from build123d import *

# Parameters (mm, degrees)
F2_R     = 12.7
F3_DEPTH = 7.62


with BuildPart() as f1:
    # F0 (on Front) → F1 (revolve)
    with BuildSketch(Plane.XZ):
        with BuildLine():
            Line((15.875, 35.306), (3.175, 35.306))
            Line((3.175, 35.306), (3.175, 0))
            Line((3.175, 0), (19.05, 0))
            Line((19.05, 0), (19.05, 3.175))
            ThreePointArc((19.05, 3.175), (16.685437, 8.304086), (15.875, 13.893529))
            Line((15.875, 13.893529), (15.875, 35.306))
        make_face()
    revolve(axis=Axis((0, 0, 26.439369), (0, 0, 1)))

    # F2 (on face) → F3 (cut)
    with BuildSketch(Plane.XY.offset(35.306)):
        Circle(F2_R)
    extrude(amount=-F3_DEPTH, mode=Mode.SUBTRACT)


solid = f1.part
Here's how the part is built. I have some questions about the finished solid (model axes, mm). A direction names the side the tool comes from. Coordinates: 2 decimals unless noted, no trailing zeros. Write each loop counter-clockwise with the first axis right and the second up, starting at its lowest first coordinate (ties: lowest second). Pieces come first, ordered by that corner, then holes.
Item 1: I want a section at C-C on z = 12. Write out the boundary of the cut face in (x, y) (3 decimals).
Item 2: If we mould it in two halves opening along Y, with no side actions, what happens to faces 3 (the flat face through (-7, 11, 35.306)), 4 (the flat face through (3, -3, 27.686)), 5 (the cylindrical face through (-3.441, -15.497, 24.75))? For each: +Y half, -Y half, draft (parallel to the pull), parting line (faces both ways), or undercut.
Item 3: If I drill on line 1 (Y direction, x = 0, z = 14) (3 decimals); line 2 (Y direction, x = 0, z = 31.75) (3 decimals); line 3 (Z direction, x = 6, y = 9), over which ranges is the centre line in solid material (lowest first)?
Item 4: On a 3-axis mill with a long thin cutter (end or side, diameter ignored), from which of +Z, -Z, +X, -X, +Y, -Y can I reach the whole of each face in a straight line? I mean faces 1 (the flat face through (-4, 0, 0)), 2 (the cylindrical face through (-2.75, -12.4, 31.55)). Say none if no direction works.
Item 5: Will these pins go through, and if not, where does the flat tip stop? pin 1 (12 mm diameter, centred on y = -4.5, z = 20, fed in from -X) (3 decimals); pin 2 (4 mm diameter, centred on x = 0.5, y = 6.5, fed in from +Z); pin 3 (6 mm diameter, centred on x = -12.5, z = 9, fed in from -Y); pin 4 (15 mm diameter, centred on x = 0, y = 0, fed in from -Z).
Item 6: I want a section at A-A on y = 0. Write out the boundary of the cut face in (x, z) (3 decimals).
Findings below:
1. outline: circle Ø31.933 at (0, 0); hole circle Ø6.35 at (0, 0)
2. face 3: draft
2. face 4: undercut
2. face 5: parting line
3. line 1: y = -15.875 to -3.175, 3.175 to 15.875
3. line 2: y = -15.875 to -12.7, 12.7 to 15.875
3. line 3: z = 0 to 27.69
4. face 1: -Z, +X, -X, +Y, -Y
4. face 2: +Z
5. pin 1: stops at x = -15.875
5. pin 2: stops at z = 27.69
5. pin 3: stops at y = -13.75
5. pin 4: stops at z = 0
6. outline: (-19.05, 0) - (-3.175, 0) - (-3.175, 27.686) - (-12.7, 27.686) - (-12.7, 35.306) - (-15.875, 35.306) - (-15.875, 13.894) arc R19.68 cw to (-19.05, 3.175) - close; (3.175, 0) - (19.05, 0) - (19.05, 3.175) arc R19.68 cw to (15.875, 13.894) - (15.875, 35.306) - (12.7, 35.306) - (12.7, 27.686) - (3.175, 27.686) - close
